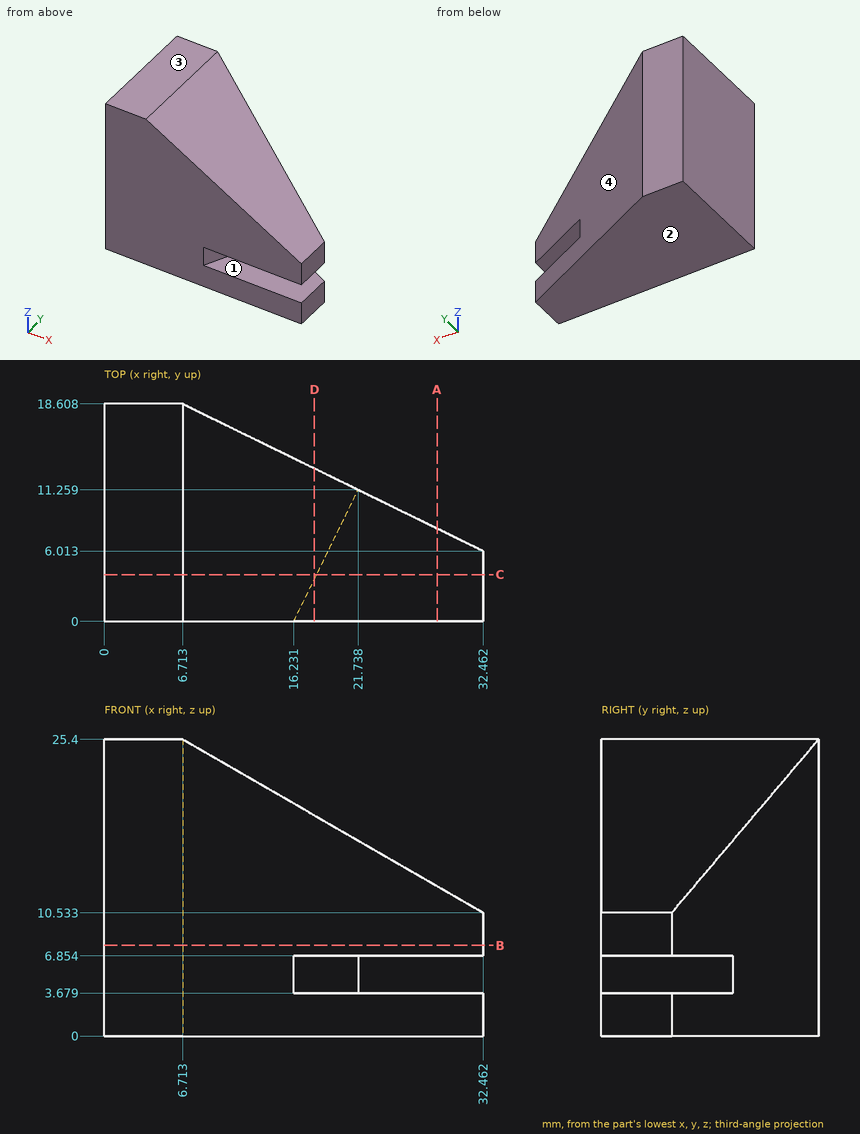
Input: dimensioned drawing with shaded views. Units: mm. Origin: part minimum x, y, z. Round coordinates to 2 decimals unless told otherwise and drop trailing zeros. Loops run counter-clockwise (first coordinate to the right, second up) from the corner with the lowest first, then second, coordinate; pieces in that order, holes last. Notation, with made-up numbers: M 53,60 L 101,60 A36 cw 101,95 Z; hole C 2,-31 d11. An arc over 180 degrees is marked long. Answer in a Markdown table with one row per item. Add a question column.
1. Ray query, probe 1 along X at (y, z) = (17.5, 16.25) (1 decimal); probe 2 along Y at (x, z) = (25, 10.75) (1 decimal); probe 3 along Z at (x, y) = (20, 12). Return the intervals inside material, ascending.
2. Section A-A (x = 28.5). Output: boundary loops of the cut face in (y, z) (1 decimal).
3. Mould query, pull axis Z, two halves, no side actions, for the marked faces 1, 2, 3 and 4. Classes: released by +Z, released by -Z, zero draft, split by the parting line, or undercut.
4. Contact query for flat-ended pins moving along their axis: pin 1 (5.5 mm diameter, centred on x = 27.5, y = 6.5, fed in from +Z) (1 decimal); pin 2 (1 mm diameter, centred on y = 9, z = 10.5, fed in from +X) (1 decimal); pin 3 (1 mm diameter, centred on x = 24, y = 8.5, fed in from +Z). Output: stop coordinate, or through.
5. Section B-B (z = 7.75). Output: boundary loops of the cut face in (x, y).
6. Section C-C (y = 4). Output: boundary loops of the cut face in (x, z) (1 decimal), and give its area (3 significant figures).
7. Section D-D (x = 18). Output: boundary loops of the cut face in (y, z) (1 decimal).
Values follow:
| question | item | result |
|---|---|---|
| 1 | probe 1 | 0 to 9 |
| 1 | probe 2 | 0 to 9.7 |
| 1 | probe 3 | 0 to 17.73 |
| 2 | outline | M 0,0 L 8,0 L 8,3.7 L 0,3.7 Z; M 0,6.9 L 8,6.9 L 8,12.8 L 0,12.8 Z |
| 3 | face 1 | undercut |
| 3 | face 2 | released by -Z |
| 3 | face 3 | released by +Z |
| 3 | face 4 | zero draft |
| 4 | pin 1 | z = 15 |
| 4 | pin 2 | x = 27.4 |
| 4 | pin 3 | z = 15.71 |
| 5 | outline | M 0,0 L 32.46,0 L 32.46,6.01 L 6.71,18.61 L 0,18.61 Z |
| 6 | outline | M 0,0 L 32.5,0 L 32.5,3.7 L 18.2,3.7 L 18.2,6.9 L 32.5,6.9 L 32.5,10.5 L 6.7,25.4 L 0,25.4 Z |
| 6 | area | 588 mm^2 |
| 7 | outline | M 0,0 L 13.1,0 L 13.1,18.9 L 0,18.9 L 0,6.9 L 3.6,6.9 L 3.6,3.7 L 0,3.7 Z |
